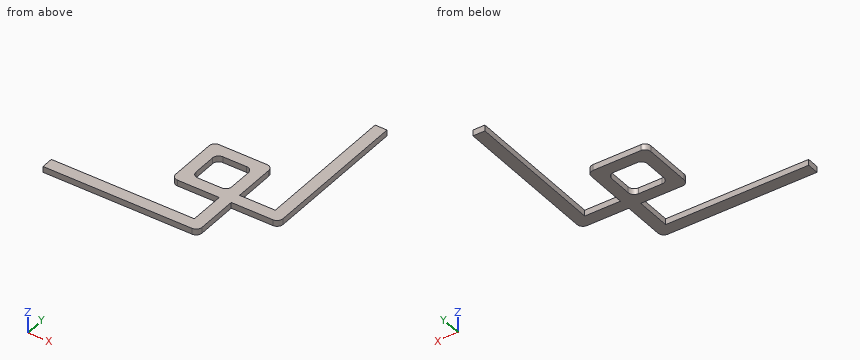
```python
from build123d import *

# Parameters (mm, degrees)
F1_DEPTH = 5


with BuildPart() as f1:
    # F0 (on Top) → F1 (new body)
    with BuildSketch(Plane.XY):
        with BuildLine():
            Line((22.006568, 31.475988), (-17.993432, 31.475988))
            ThreePointArc((-17.993432, 31.475988), (-21.528966, 30.011522), (-22.993432, 26.475988))
            Line((-22.993432, 26.475988), (-22.993432, -13.524012))
            ThreePointArc((-22.993432, -13.524012), (-21.528966, -17.059546), (-17.993432, -18.524012))
            Line((-17.993432, -18.524012), (17.006568, -18.524012))
            Line((17.006568, -18.524012), (27.006568, -18.524012))
            Line((27.006568, -18.524012), (27.006568, -8.524012))
            Line((27.006568, -8.524012), (27.006568, 26.475988))
            ThreePointArc((27.006568, 26.475988), (25.542101, 30.011522), (22.006568, 31.475988))
        make_face()
        with BuildLine():
            ThreePointArc((-12.993432, 16.475988), (-11.528966, 20.011522), (-7.993432, 21.475988))
            Line((-7.993432, 21.475988), (12.006568, 21.475988))
            ThreePointArc((12.006568, 21.475988), (15.542101, 20.011522), (17.006568, 16.475988))
            Line((17.006568, 16.475988), (17.006568, -3.524012))
            ThreePointArc((17.006568, -3.524012), (15.542101, -7.059546), (12.006568, -8.524012))
            Line((12.006568, -8.524012), (-7.993432, -8.524012))
            ThreePointArc((-7.993432, -8.524012), (-11.528966, -7.059546), (-12.993432, -3.524012))
            Line((-12.993432, -3.524012), (-12.993432, 16.475988))
        make_face(mode=Mode.SUBTRACT)
        with BuildLine():
            Line((57.006568, -8.524012), (27.006568, -8.524012))
            Line((27.006568, -8.524012), (27.006568, -18.524012))
            Line((27.006568, -18.524012), (62.006568, -18.524012))
            ThreePointArc((62.006568, -18.524012), (65.542101, -17.059546), (67.006568, -13.524012))
            Line((67.006568, -13.524012), (67.006568, 111.475988))
            Line((67.006568, 111.475988), (57.006568, 111.475988))
            Line((57.006568, 111.475988), (57.006568, -8.524012))
        make_face()
        with BuildLine():
            Line((27.006568, -53.524012), (27.006568, -18.524012))
            Line((27.006568, -18.524012), (17.006568, -18.524012))
            Line((17.006568, -18.524012), (17.006568, -48.524012))
            Line((17.006568, -48.524012), (-102.993432, -48.524012))
            Line((-102.993432, -48.524012), (-102.993432, -58.524012))
            Line((-102.993432, -58.524012), (22.006568, -58.524012))
            ThreePointArc((22.006568, -58.524012), (25.542101, -57.059546), (27.006568, -53.524012))
        make_face()
    extrude(amount=F1_DEPTH)


solid = f1.part
```
Can you work these out from the model? Positions are in its coordinate system, mm. Round coordinates to 2 decimals unless told otherwise and drop trailing zeros. Loops run counter-clockwise (first coordinate to the right, second up) from the corner with the lowest first, then second, coordinate; pieces in that order, holes last. Notation, with made-up numbers: (-37.75, 86) -> (-3.75, 86) arc R8 ccw to (-3.75, 91) -> close; hole circle Ø8 at (-38.5, 86). An arc over 180 degrees is marked (long way). One line per item, written item: value. Start each with the question number.
1. If we section it at B-B, the plane x = -16: Write out the boundary of the cut face in (y, z).
2. If we section it at D-D, the plane y = 94: Write out the boundary of the cut face in (x, z), then the cut area to 3 significant figures.
3. If we section it at A-A, the plane x = 9: Write out the boundary of the cut face in (y, z).
4. If I drill on probe 1 along X at (y, z) = (3.5, 3.85); probe 2 along Y at (x, z) = (-1.5, 0.25); probe 3 along X at (y, z) = (22, 2.3), over which ranges is the centre line in solid material (lowest first)?
5. For pin 1 (1.5 mm diameter, centred on x = -4.5, z = 2, fed in from +Y); pin 2 (2.5 mm diameter, centred on y = -2.5, z = 3.5, fed in from -X); pin 3 (1 mm diameter, centred on x = -57.5, z = 2, fed in from +Y), each with a flat end and sliding along its axis, tell me the tip position at first contact or that it passes through.
6. If we section it at C-C, the plane z = 3.05: Write out the boundary of the cut face in (x, y), then the cut area to 3 significant figures.
Calculated:
1. outline: (-58.52, 0) -> (-48.52, 0) -> (-48.52, 5) -> (-58.52, 5) -> close; (-18.52, 0) -> (31.48, 0) -> (31.48, 5) -> (-18.52, 5) -> close
2. outline: (57.01, 0) -> (67.01, 0) -> (67.01, 5) -> (57.01, 5) -> close
2. area: 50.0 mm²
3. outline: (-58.52, 0) -> (-48.52, 0) -> (-48.52, 5) -> (-58.52, 5) -> close; (-18.52, 0) -> (-8.52, 0) -> (-8.52, 5) -> (-18.52, 5) -> close; (21.48, 0) -> (31.48, 0) -> (31.48, 5) -> (21.48, 5) -> close
4. probe 1: x = -22.99 to -12.99, 17.01 to 27.01, 57.01 to 67.01
4. probe 2: y = -58.52 to -48.52, -18.52 to -8.52, 21.48 to 31.48
4. probe 3: x = -22.99 to 27.01, 57.01 to 67.01
5. pin 1: stops at y = 31.48
5. pin 2: stops at x = -22.99
5. pin 3: stops at y = -48.52
6. outline: (-102.99, -58.52) -> (22.01, -58.52) arc R5 ccw to (27.01, -53.52) -> (27.01, -18.52) -> (62.01, -18.52) arc R5 ccw to (67.01, -13.52) -> (67.01, 111.48) -> (57.01, 111.48) -> (57.01, -8.52) -> (27.01, -8.52) -> (27.01, 26.48) arc R5 ccw to (22.01, 31.48) -> (-17.99, 31.48) arc R5 ccw to (-22.99, 26.48) -> (-22.99, -13.52) arc R5 ccw to (-17.99, -18.52) -> (17.01, -18.52) -> (17.01, -48.52) -> (-102.99, -48.52) -> close; hole (-12.99, -3.52) arc R5 ccw to (-7.99, -8.52) -> (12.01, -8.52) arc R5 ccw to (17.01, -3.52) -> (17.01, 16.48) arc R5 ccw to (12.01, 21.48) -> (-7.99, 21.48) arc R5 ccw to (-12.99, 16.48) -> close
6. area: 4,790 mm²
